```python
from build123d import *

# Parameters (mm, degrees)
SKETCH_1_W          = 22
SKETCH_1_H          = 22
SKETCH_1_R          = 6
EXTRUDE_1_DEPTH     = 5
SKETCH_3_OUTSIDE_W  = 30.302
SKETCH_3_OUTSIDE_H  = 30.302
SKETCH_3_OUTSIDE_R  = 14
CUT_EXTRUDE_2_DEPTH = 5
SKETCH_5_R          = 1.75
CUT_EXTRUDE_3_DEPTH = 5
SKETCH_5_3_R        = 3
SKETCH_5_3_R_2      = 1.75
CUT_EXTRUDE_4_DEPTH = 3.1
CHAMFER_1_SIZE      = 0.1
SKETCH_7_R          = 6
SKETCH_7_R_2        = 5.5
EXTRUDE_2_DEPTH     = 19
FILLET_1_R          = 0.2
CHAMFER_2_SIZE      = 0.1
FILLET_2_R          = 0.1


with BuildPart() as part:
    # Sketch 1 → Extrude 1 (new body)
    with BuildSketch(Plane.XY):
        Rectangle(SKETCH_1_W, SKETCH_1_H)
        Circle(SKETCH_1_R, mode=Mode.SUBTRACT)
    extrude(amount=EXTRUDE_1_DEPTH)

    # Sketch 3 outside → Cut-Extrude 2 (cut)
    with BuildSketch(Plane.XY.offset(5)):
        Rectangle(SKETCH_3_OUTSIDE_W, SKETCH_3_OUTSIDE_H)
        Circle(SKETCH_3_OUTSIDE_R, mode=Mode.SUBTRACT)
    extrude(amount=-CUT_EXTRUDE_2_DEPTH, mode=Mode.SUBTRACT)

    # Sketch 5 → Cut-Extrude 3 (cut)
    with BuildSketch(Plane.XY):
        with Locations(Location((-7.071067812, 7.071067812, 0), (0, 0, 180))):  # turned: the seam where the file's is
            Circle(SKETCH_5_R)
        with Locations(Location((-7.071067812, -7.071067812, 0), (0, 0, 180))):  # turned: the seam where the file's is
            Circle(SKETCH_5_R)
        with Locations(Location((7.071067812, -7.071067812, 0), (0, 0, 180))):  # turned: the seam where the file's is
            Circle(SKETCH_5_R)
        with Locations(Location((7.071067812, 7.071067812, 0), (0, 0, 180))):  # turned: the seam where the file's is
            Circle(SKETCH_5_R)
    extrude(amount=CUT_EXTRUDE_3_DEPTH, mode=Mode.SUBTRACT)

    # Sketch 5_3 → Cut-Extrude 4 (cut)
    with BuildSketch(Plane.XY):
        with Locations((-7.071067812, 7.071067812)):
            Circle(SKETCH_5_3_R)
        with Locations(Location((-7.071067812, 7.071067812, 0), (0, 0, 180))):  # turned: the seam where the file's is
            Circle(SKETCH_5_3_R_2, mode=Mode.SUBTRACT)
        with Locations(Location((7.071067812, 7.071067812, 0), (0, 0, 180))):  # turned: the seam where the file's is
            Circle(SKETCH_5_3_R)
        with Locations(Location((7.071067812, 7.071067812, 0), (0, 0, 180))):  # turned: the seam where the file's is
            Circle(SKETCH_5_3_R_2, mode=Mode.SUBTRACT)
        with Locations((7.071067812, -7.071067812)):
            Circle(SKETCH_5_3_R)
        with Locations(Location((7.071067812, -7.071067812, 0), (0, 0, 180))):  # turned: the seam where the file's is
            Circle(SKETCH_5_3_R_2, mode=Mode.SUBTRACT)
        with Locations(Location((-7.071067812, -7.071067812, 0), (0, 0, 180))):  # turned: the seam where the file's is
            Circle(SKETCH_5_3_R)
        with Locations(Location((-7.071067812, -7.071067812, 0), (0, 0, 180))):  # turned: the seam where the file's is
            Circle(SKETCH_5_3_R_2, mode=Mode.SUBTRACT)
    extrude(amount=CUT_EXTRUDE_4_DEPTH, mode=Mode.SUBTRACT)

    # Chamfer 1
    chamfer_1_edges = [part.edges().sort_by_distance(p)[0] for p in [
        (10.071067812, 7.071067812, 0),
        (-10.071067812, 7.071067812, 0),
        (-6, 0, 0),
        (-6, 0, 5),
        (0, -11, 0),
        (0, -11, 5),
        (-11, 0, 0),
        (-11, 0, 5),
        (0, 11, 0),
        (0, 11, 5),
        (11, 0, 0),
        (11, 0, 5),
        (9.899494937, -9.899494937, 5),
        (9.899494937, 9.899494937, 5),
        (-9.899494937, 9.899494937, 5),
        (-9.899494937, -9.899494937, 5),
        (9.899494937, 9.899494937, 0),
        (-9.899494937, 9.899494937, 0),
        (9.899494937, -9.899494937, 0),
        (-9.899494937, -9.899494937, 0),
        (8.821067812, 7.071067812, 5),
        (8.821067812, -7.071067812, 5),
        (-5.321067812, -7.071067812, 5),
        (-5.321067812, 7.071067812, 5),
        (-4.071067812, -7.071067812, 0),
        (4.071067812, -7.071067812, 0),
    ]]
    chamfer(chamfer_1_edges, length=CHAMFER_1_SIZE)

    # Sketch 7 → Extrude 2 (add)
    with BuildSketch(Plane(origin=(0, 0, 0), x_dir=(-1, 0, 0), z_dir=(0, 0, -1))):
        Circle(SKETCH_7_R)
        Circle(SKETCH_7_R_2, mode=Mode.SUBTRACT)
    extrude(amount=-EXTRUDE_2_DEPTH)

    # Fillet 1
    fillet_1_edges = [part.edges().sort_by_distance(p)[0] for p in [
        (6, 0, 19),
    ]]
    fillet(fillet_1_edges, radius=FILLET_1_R)

    # Chamfer 2
    chamfer_2_edges = [part.edges().sort_by_distance(p)[0] for p in [
        (5.5, 0, 19),
    ]]
    chamfer(chamfer_2_edges, length=CHAMFER_2_SIZE)

    # Sketch 8 → Revolve 1 (revolve)
    with BuildSketch(Plane(origin=(0, 0, 0), x_dir=(0, 0, -1), z_dir=(1, 0, 0)), mode=Mode.PRIVATE) as revolve_1_sk:
        Polygon((-18.5, 5.5), (-0.4, 5.5), (-0.4, 5.3), (-0.2, 5.3), (-0.2, 3.3), (0, 3.3), (0, 3), (-0.693888948, 3), (-18.206111052, 3), (-18.9, 3), (-18.9, 3.3), (-18.7, 3.3), (-18.7, 5.3), (-18.5, 5.3), align=None)
    revolve(revolve_1_sk.sketch.rotate(Axis((0, 0, 0), (0, 0, 1)), 90), axis=Axis((0, 0, 0), (0, 0, 1)))  # turned: the seam where the file's is

    # Fillet 2
    fillet_2_edges = [part.edges().sort_by_distance(p)[0] for p in [
        (-8.660254038, 11, 2.5),
        (-11, 8.660254038, 2.5),
        (-11, -8.660254038, 2.5),
        (-8.660254038, -11, 2.5),
        (8.660254038, -11, 2.5),
        (11, -8.660254038, 2.5),
        (11, 8.660254038, 2.5),
        (8.660254038, 11, 2.5),
    ]]
    fillet(fillet_2_edges, radius=FILLET_2_R)


solid = part.part
```
Geometry check sheet. Reference: the model listing, model coordinates, mm. A direction names the side the tool comes from. Give positions to 0.01 mm unless a question says otherwise; leave off trailing zeros. Order: outer loops, then holes, each group sorted by start corner. A loop starts at its lowest first (then second) coordinate and runs counter-clockwise, first axis right, second up.
1. Thickness scan on L1, parallel to X at y = 8.75, z = 1.75; L2, parallel to X at y = 0.5, z = 6; L3, parallel to Z at x = 5.5, y = -3. Record the ranges inside material, lowest first.
2. Section check B-B, the plane z = 6. Enter the section's corners in (x, y), and give its area (3 significant figures).
3. Access from +Z, -Z, +X, -X, +Y, -Y to the whole of each face (thin tool, end or side, straight path). Record for faces 1 (the face through (-9, -7, 3.1)), 2 (the face through (-5.682, 8.136, 3.987)).
4. Section check A-A, the plane z = 2. Enter the section's corners in (x, y), and give its area (3 significant figures).
5. Release check for a two-part mould opening along Y. For faces 3 (the face through (0, -11, 2)), 4 (the face through (-3, -5, 0)), 5 (the face through (-5.46, 9.6, 1.58)), 6 (the face through (-5.78, -8.25, 3.99)) record: pulls with the +Y half, pulls with the -Y half, needs draft (parallel to the pull), parting line crosses it, or undercut.
6. Gauge pin test, flat ends, axial feed: pin 1 Ø4.5 at (x, y) = (7.07, 7.07) entering from +Z; pin 2 Ø3 at (x, y) = (6.5, 7) entering from -Z; pin 3 Ø2 at (y, z) = (-4, 11.5) entering from -X. Record the tip position at first contact, or that the pin passes through.
Values follow:
1. L1: x = -10.93 to -9.56, -4.58 to 4.58, 9.56 to 10.93
1. L2: x = -5.98 to -2.96, 2.96 to 5.98
1. L3: z = 0 to 5
2. outline: circle Ø12 at (0, 0); hole circle Ø6 at (0, 0)
2. area: 84.8 mm2
3. face 1: -Z
3. face 2: +Z, -Z
4. outline: (-11, -8.63) arc R0.1 ccw to (-10.98, -8.69) arc R14 ccw to (-8.69, -10.98) arc R0.1 ccw to (-8.63, -11) - (8.63, -11) arc R0.1 ccw to (8.69, -10.98) arc R14 ccw to (10.98, -8.69) arc R0.1 ccw to (11, -8.63) - (11, 8.63) arc R0.1 ccw to (10.98, 8.69) arc R14 ccw to (8.69, 10.98) arc R0.1 ccw to (8.63, 11) - (-8.63, 11) arc R0.1 ccw to (-8.69, 10.98) arc R14 ccw to (-10.98, 8.69) arc R0.1 ccw to (-11, 8.63) - close; hole circle Ø6 at (-7.07, -7.07); hole circle Ø6 at (-7.07, 7.07); hole circle Ø6 at (0, 0); hole circle Ø6 at (7.07, -7.07); hole circle Ø6 at (7.07, 7.07)
4. area: 333 mm2
5. face 3: pulls with the -Y half
5. face 4: needs draft
5. face 5: undercut
5. face 6: undercut
6. pin 1: stops at z = 5
6. pin 2: stops at z = 3.1
6. pin 3: stops at x = -5.2
